Input: part model. Units: mm. Frame: model coordinates. A direction names the side the tool comes from. Round coordinates to 2 decimals unless told otherwise and drop trailing zeros. Loops run counter-clockwise (first coordinate to the right, second up) from the corner with the lowest first, then second, coordinate; pieces in that order, holes last. Notation, with made-up numbers: (-18.5, -12.5) -> (16.5, -12.5) arc R18 cw to (16.5, 7.5) -> close; hole circle Ø4 at (62.5, 22). An arc over 180 degrees is marked (long way). Answer as a JSON object with one key per item and string values.
```python
from build123d import *

# Parameters (mm, degrees)
F0_R            = 135
F1_DEPTH        = 3
F3_D            = 4
F3_COPIES_COUNT = 6


# Not quite as in the source:
# - a pattern or mirror of a feature is missing from the dataset's text; its kind, count and spacing are read off the source's solid


with BuildPart() as f1:
    # F0 (on Front) → F1 (new body)
    with BuildSketch(Plane.XZ):
        Circle(F0_R)
        with BuildLine():
            Line((-78.968744185, -57.1396310965), (-32.3120288915, -30.2023639624))
            ThreePointArc((-32.3120288915, -30.2023639624), (-26.8672094621, -28.8725161151), (-21.5621280722, -30.6810142107))
            ThreePointArc((-21.5621280722, -30.6810142107), (0, -37.5), (21.5621280722, -30.6810142107))
            ThreePointArc((21.5621280722, -30.6810142107), (26.8672094621, -28.8725161151), (32.3120288915, -30.2023639624))
            Line((32.3120288915, -30.2023639624), (78.968744185, -57.1396310965))
            ThreePointArc((78.968744185, -57.1396310965), (83.8408747407, -64.2058216819), (81.4403345067, -72.4463381783))
            ThreePointArc((81.4403345067, -72.4463381783), (0, -109), (-81.4403345067, -72.4463381783))
            ThreePointArc((-81.4403345067, -72.4463381783), (-83.8408747407, -64.2058216819), (-78.968744185, -57.1396310965))
        make_face(mode=Mode.SUBTRACT)
        with BuildLine():
            ThreePointArc((-10, 43.084219849), (-11.5707276958, 37.7039439805), (-15.7894736842, 34.0138577756))
            ThreePointArc((-15.7894736842, 34.0138577756), (-32.4759526419, 18.75), (-37.3516017564, -3.3328435649))
            ThreePointArc((-37.3516017564, -3.3328435649), (-38.4379371579, -8.8314278655), (-42.3120288915, -12.8818558867))
            Line((-42.3120288915, -12.8818558867), (-88.968744185, -39.8191230209))
            ThreePointArc((-88.968744185, -39.8191230209), (-97.5243100178, -40.50541656), (-103.4605365269, -34.3062294864))
            ThreePointArc((-103.4605365269, -34.3062294864), (-94.3967690125, 54.5), (-22.0202020202, 106.7525676646))
            ThreePointArc((-22.0202020202, 106.7525676646), (-13.6834352771, 104.7112382419), (-10, 96.9587541174))
            Line((-10, 96.9587541174), (-10, 43.084219849))
        make_face(mode=Mode.SUBTRACT)
        with BuildLine():
            ThreePointArc((15.7894736842, 34.0138577756), (11.5707276958, 37.7039439805), (10, 43.084219849))
            Line((10, 43.084219849), (10, 96.9587541174))
            ThreePointArc((10, 96.9587541174), (13.6834352771, 104.7112382419), (22.0202020202, 106.7525676646))
            ThreePointArc((22.0202020202, 106.7525676646), (94.3967690125, 54.5), (103.4605365269, -34.3062294864))
            ThreePointArc((103.4605365269, -34.3062294864), (97.5243100178, -40.50541656), (88.968744185, -39.8191230209))
            Line((88.968744185, -39.8191230209), (42.3120288915, -12.8818558867))
            ThreePointArc((42.3120288915, -12.8818558867), (38.4379371579, -8.8314278655), (37.3516017564, -3.3328435649))
            ThreePointArc((37.3516017564, -3.3328435649), (32.4759526419, 18.75), (15.7894736842, 34.0138577756))
        make_face(mode=Mode.SUBTRACT)
    extrude(amount=F1_DEPTH)

    # F3 (through all)
    with Locations(Plane(origin=(0, 0, 0), x_dir=(1, 0, 0), z_dir=(0, 1, 0))):
        with Locations((0, -25)):
            f3 = Hole(F3_D / 2)

    # F3_copies: F3 ×6 about axis
    f3_copies_axis = Axis((0, 0, 0), (0, 1, 0))
    for i in range(1, F3_COPIES_COUNT):
        add(f3.rotate(f3_copies_axis, i * 360 / F3_COPIES_COUNT), mode=Mode.SUBTRACT)


solid = f1.part
```
1) Ray query, probe 1 along Z at (x, y) = (0, -2.3); probe 2 along Z at (x, y) = (78, -1.9); probe 3 along Z at (x, y) = (-82.5, -2.35). Return the intervals inside material, ascending.
Output:
{"probe 1": "z = -135 to -109, -37.5 to -27, -23 to 23, 27 to 135", "probe 2": "z = -110.19 to -76.14, -56.58 to -33.49, 76.14 to 110.19", "probe 3": "z = -106.86 to -71.02, -60.58 to -36.08, 71.24 to 106.86"}
2) Reachability of faces 4 (the face through (32.636, -1.479, 18.471)), 5 (the face through (-2, -3, 2)) from +Z, -Z, +X, -X, +Y, -Y: full face, straight path, thin tool, end or side. Return the list, or none.
Output:
{"face 4": "+Y, -Y", "face 5": "+Z, -Z, +X, -X, -Y"}
3) Contact query for flat-ended pins moving along their axis: P1, Ø6.5, axis at x = 21.65, z = 12.5, coming from the +Y side; P2, Ø1.5, axis at y = -1, z = 63.5, coming from the -X side. Output: stop coordinate, or through.
Output:
{"P1": "stops at y = 0", "P2": "stops at x = -119.53"}
4) Section D-D, the plane x = -57.5. Output: boundary loops of the cut face in (y, z).
Output:
{"outline": "(-3, -122.14) -> (0, -122.14) -> (0, -92.6) -> (-3, -92.6) -> close; (-3, -44.74) -> (0, -44.74) -> (0, -21.65) -> (-3, -21.65) -> close; (-3, 92.6) -> (0, 92.6) -> (0, 122.14) -> (-3, 122.14) -> close"}
5) Section A-A, the plane z = -48.5. Output: boundary loops of the cut face in (x, y).
Output:
{"outline": "(-125.99, -3) -> (-64, -3) -> (-64, 0) -> (-125.99, 0) -> close; (64, -3) -> (125.99, -3) -> (125.99, 0) -> (64, 0) -> close"}
6) Draft query along X for faces 1 (the face through (1.288, -1.479, -108.992)), 2 (the face through (-107.13, -1.48, -82.15)), 3 (the face through (-2, 0, 2)). Return one class per face: +X half, -X half, draft (parallel to the pull), parting line (faces both ways), or undercut.
Output:
{"face 1": "undercut", "face 2": "parting line", "face 3": "draft"}
7) Section C-C, the plane y = -2.5. Count the separate pieces of the cut face and the enclosed holes in it, plus the area to 3 significant figures.
Output:
{"separate pieces": "1", "enclosed holes": "9", "area": "28,800 mm^2"}
8) Section B-B, the plane x = 50.5. Output: boundary loops of the cut face in (y, z).
Output:
{"outline": "(-3, -125.2) -> (0, -125.2) -> (0, -96.6) -> (-3, -96.6) -> close; (-3, -40.7) -> (0, -40.7) -> (0, -17.61) -> (-3, -17.61) -> close; (-3, 96.6) -> (0, 96.6) -> (0, 125.2) -> (-3, 125.2) -> close"}
